Design review of the part shown in the three views and the two pictorial views. Dimensions are in mm from the part's minimum x, y and z. Give positions to 0.01 mm unless a question says otherwise; leave off trailing zeros. Order: outer loops, then holes, each group sorted by start corner. A loop starts at its lowest first (then second) coordinate and runs counter-clockwise, first axis right, second up. Notation, with made-up numbers: (74.25, 57) - (121.25, 57) arc R20 ccw to (121.25, 66) - close; hole circle Ø6 at (78, 4.5). An arc over 180 degrees is marked (long way). Put each result on its own line as item: value. Start each with the question number.
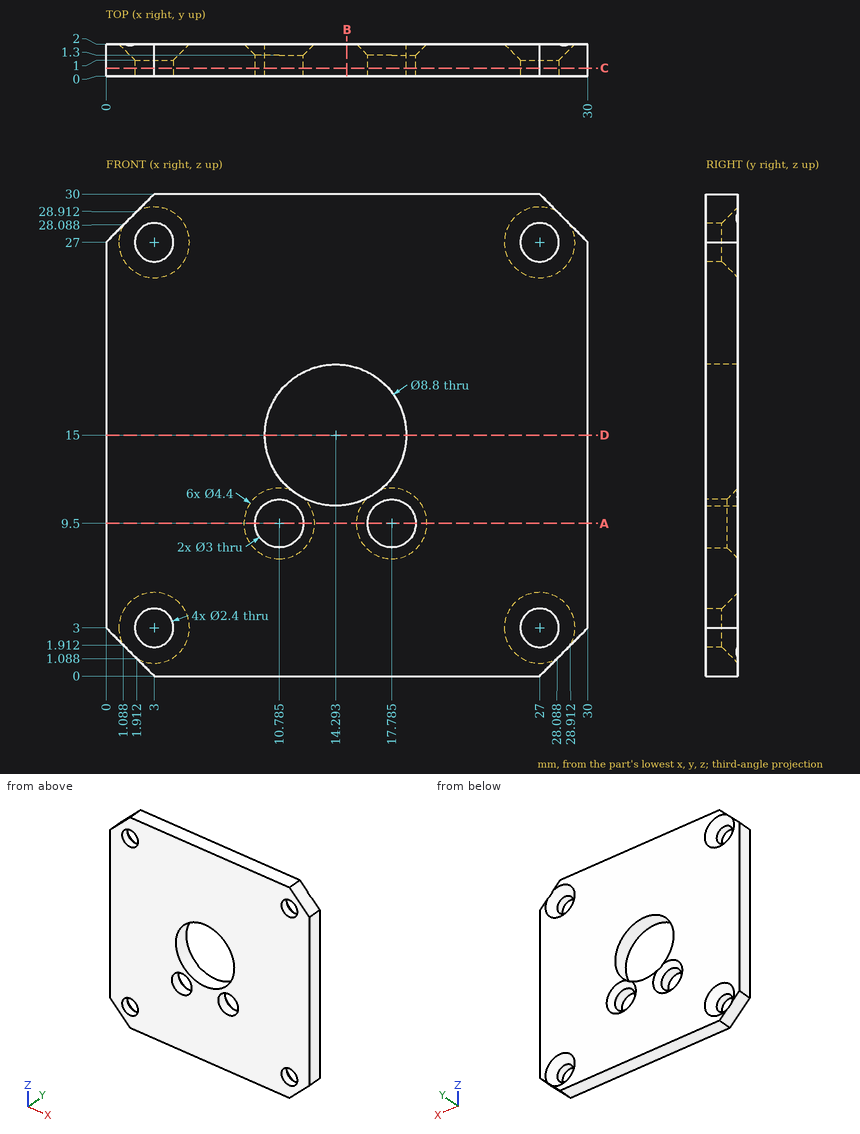
1. Add section B-B, the plane x = 15. Give the boundary of the cut face in (y, z).
2. Add section A-A, the plane z = 9.5. Give the boundary of the cut face in (x, y) (1 decimal).
3. Add section C-C, the plane y = 0.5. Give the boundary of the cut face in (x, z) (1 decimal).
4. Wall thickness on line 1 (X direction, y = 0.5, z = 27); line 2 (X direction, y = 0.3, z = 14.75): over which ranges is each line inside the solid? List them lowest first. Write a range as from..to.
5. Add section D-D, the plane z = 15. Give the boundary of the cut face in (x, y), then the cut area to 3 significant figures.
6. Clearance check with flat-ended pins moving along their axes: pin 1 (3.5 mm diameter, centred on x = 10.78, z = 9.5, fed in from +Y) (1 decimal); pin 2 (2 mm diameter, centred on x = 3, z = 27, fed in from -Y); pin 3 (3 mm diameter, centred on x = 27, z = 3, fed in from +Y). State where each tip first meets the part, or that it passes through.
Found:
1. outline: (0, 0) - (2, 0) - (2, 10.66) - (0, 10.66) - close; (0, 19.34) - (2, 19.34) - (2, 30) - (0, 30) - close
2. outline: (0, 0) - (9.3, 0) - (9.3, 1.3) - (8.6, 2) - (0, 2) - close; (12.3, 0) - (16.3, 0) - (16.3, 1.3) - (15.6, 2) - (13, 2) - (12.3, 1.3) - close; (19.3, 0) - (30, 0) - (30, 2) - (20, 2) - (19.3, 1.3) - close
3. outline: (0, 3) - (3, 0) - (27, 0) - (30, 3) - (30, 27) - (27, 30) - (3, 30) - (0, 27) - close; hole circle Ø2.4 at (3, 3); hole circle Ø2.4 at (3, 27); hole circle Ø3 at (10.8, 9.5); hole circle Ø8.8 at (14.3, 15); hole circle Ø3 at (17.8, 9.5); hole circle Ø2.4 at (27, 3); hole circle Ø2.4 at (27, 27)
4. line 1: x = 0..1.8, 4.2..25.8, 28.2..30
4. line 2: x = 0..9.9, 18.69..30
5. outline: (0, 0) - (9.89, 0) - (9.89, 2) - (0, 2) - close; (18.69, 0) - (30, 0) - (30, 2) - (18.69, 2) - close
5. area: 42.4 mm^2
6. pin 1: stops at y = 1.6
6. pin 2: passes through
6. pin 3: stops at y = 1.3
